Build history of the part. All positions in model axes, mm. A direction names the side the tool comes from. Coordinates: 2 decimals unless noted, no trailing zeros. Loops run counter-clockwise (first coordinate to the right, second up) from the corner with the lowest first, then second, coordinate; pieces in that order, holes last.
(1) Slice it at A-A (z = -1). Give the cut face in (x, y), and give its area (3 significant figures).
(2) Slice it at D-D (x = 10). Give the cut face in (y, z).
(3) Tool access for faces 1 (the face through (15, 2, -28)), 2 (the face through (20, 1, -11.25)), 3 (the face through (16.845, 4.522, -9.03)): list every direction of +Z, -Z, +X, -X, +Y, -Y with a clear straight run to the whole face (end or side of a thin tool).
(4) Two-plate mould, pull along X, no slides. Class faces 4 (the face through (-11.22, 2.74, -8.78)), 5 (the face through (22.25, 1, -9)), 6 (the face through (-16, 4, 11.25)): pulls with the +X half, pulls with the -X half, needs draft (parallel to the pull), parting line crosses it, or undercut.
(5) Wall check: L1, parallel to X at y = 3.55, z = -27.5; L2, parallel to X at y = 0.75, z = -18.5; L3, parallel to X at y = 4.25, z = -9. Give the ranges that are in metal, low to high.
(6) Slice it at B-B (y = 0.75). Give the cut face in (x, z), and give its area (4 significant figures).
(7) Flat gauge pins, fed straight in: P1, Ø1.5, axis at x = -13.5, y = 3.5, coming from the +Z side; P2, Ø2, axis at y = 2.5, z = -2, coming from the -X side; P3, Ø1.8, axis at x = 20, y = 1, coming from the -Z side; P4, Ø1.5, axis at x = 4, z = -8.5, coming from the +Y side. Where does each tip first touch, or does it go through?
(8) Slice it at C-C (x = -7.5). Give the cut face in (y, z).
from build123d import *

# Parameters (mm, degrees)
SKETCH_1_W          = 4
SKETCH_1_H          = 17.5
SKETCH_1_H_2        = 5
EXTRUDE_1_DEPTH     = 4
SKETCH_1_7_W        = 44.5
SKETCH_1_7_H        = 5
EXTRUDE_2_DEPTH     = 3.5
SKETCH_2_W          = 18.5
SKETCH_2_H          = 1.5
CUT_EXTRUDE_1_DEPTH = 32.89533665
SKETCH_2_3_W        = 2.5
SKETCH_2_3_H        = 1.5
EXTRUDE_4_DEPTH     = 22.5
FILLET_1_R          = 1
FILLET_2_R          = 1.5
FILLET_3_R          = 1
SKETCH_5_W          = 2.5
SKETCH_5_H          = 2
CUT_EXTRUDE_2_DEPTH = 43.315038698
SKETCH_10_R         = 0.4
CUT_EXTRUDE_3_DEPTH = 2


with BuildPart() as part:
    # 草图1 → 凸台-拉伸1 (new body)
    with BuildSketch(Plane(origin=(0, 0, 0), x_dir=(1, 0, 0), z_dir=(0, 1, 0))):
        with Locations((-15.75, -2.5)):
            Rectangle(SKETCH_1_W, SKETCH_1_H)
        with Locations((15.75, -2.5)):
            Rectangle(SKETCH_1_W, SKETCH_1_H)
        with Locations((15.75, 8.75)):
            Rectangle(SKETCH_1_W, SKETCH_1_H_2)
        with Locations((-15.75, 8.75)):
            Rectangle(SKETCH_1_W, SKETCH_1_H_2)
    extrude(amount=EXTRUDE_1_DEPTH)

    # 草图1<7> → 凸台-拉伸2 (add)
    with BuildSketch(Plane(origin=(0, 0, 0), x_dir=(1, 0, 0), z_dir=(0, 1, 0))):
        with Locations((0, 8.75)):
            Rectangle(SKETCH_1_7_W, SKETCH_1_7_H)
    extrude(amount=EXTRUDE_2_DEPTH)

    # 草图2 → 切除-拉伸1 (cut, through all)
    with BuildSketch(Plane(origin=(0, 0, -11.25), x_dir=(-1, 0, 0), z_dir=(0, 0, -1))):
        with Locations((0, 2.75)):
            Rectangle(SKETCH_2_W, SKETCH_2_H)
        Polygon((13.25, 3.5), (9.25, 3.5), (9.25, 2), align=None)
        Polygon((-9.25, 3.5), (-13.25, 3.5), (-9.25, 2), align=None)
        Polygon((-22.25, 3.5), (-22.25, 2), (-18.25, 3.5), align=None)
        Polygon((22.25, 3.5), (18.25, 3.5), (22.25, 2), align=None)
    extrude(amount=-CUT_EXTRUDE_1_DEPTH, mode=Mode.SUBTRACT)

    # 草图2<3> → 凸台-拉伸4 (add, through all)
    with BuildSketch(Plane(origin=(0, 0, -11.25), x_dir=(-1, 0, 0), z_dir=(0, 0, -1))):
        with Locations((-15.75, 7.25)):
            Rectangle(SKETCH_2_3_W, SKETCH_2_3_H)
        Polygon((-15, 6.5), (-16.5, 6.5), (-16.5, 4), (-15.75, 4), (-15, 4), align=None)
        with Locations((15.75, 7.25)):
            Rectangle(SKETCH_2_3_W, SKETCH_2_3_H)
        Polygon((16.5, 6.5), (15, 6.5), (15, 4), (15.75, 4), (16.5, 4), align=None)
    extrude(amount=-EXTRUDE_4_DEPTH)

    # 圆角1
    # the kernel refuses this fillet: 1 mm, written as the material it adds along each edge
    with BuildSketch(Plane(origin=(-16.5, 6.5, -11.25), x_dir=(0, -1, 0), z_dir=(0, 0, 1))) as fillet_1_piece_1:
        with BuildLine():
            CenterArc((0.866025404, -1), FILLET_1_R, 90, 60)
            Line((0, -0.5), (-0.017320508, -0.49))
            ThreePointArc((-0.017320508, -0.49), (-0.02, -0.25), (-0.02, 0))
            Line((-0.02, 0), (0, 0.02))
            Line((0, 0.02), (0.866025404, 0.02))
            Line((0.866025404, 0.02), (0.866025404, 0))
        make_face()
    extrude(amount=22.5)
    with BuildSketch(Plane(origin=(-15, 6.5, -11.25), x_dir=(0, -1, 0), z_dir=(0, 0, 1)), Plane(origin=(16.5, 6.5, -11.25), x_dir=(0, -1, 0), z_dir=(0, 0, 1))) as fillet_1_piece_2:
        with BuildLine():
            CenterArc((0.866025404, 1), FILLET_1_R, 210, 60)
            Line((0, 0.5), (-0.017320508, 0.49))
            ThreePointArc((-0.017320508, 0.49), (-0.02, 0.25), (-0.02, 0))
            Line((-0.02, 0), (0, -0.02))
            Line((0, -0.02), (0.866025404, -0.02))
            Line((0.866025404, -0.02), (0.866025404, 0))
        make_face()
    extrude(amount=22.5)
    with BuildSketch(Plane(origin=(15, 6.5, -11.25), x_dir=(-1, 0, 0), z_dir=(0, 0, 1))) as fillet_1_piece_3:
        with BuildLine():
            CenterArc((1, 0.866025404), FILLET_1_R, 180, 60)
            Line((0, 0.866025404), (-0.02, 0.866025404))
            Line((-0.02, 0.866025404), (-0.02, 0))
            Line((-0.02, 0), (0, -0.02))
            ThreePointArc((0, -0.02), (0.25, -0.02), (0.49, -0.017320508))
            Line((0.49, -0.017320508), (0.5, 0))
        make_face()
    extrude(amount=22.5)

    # 圆角2
    # the kernel refuses this fillet: 1.5 mm, written as the material it adds along each edge
    with BuildSketch(Plane(origin=(16.5, 4, -11.25), x_dir=(1, 0, 0), z_dir=(0, 0, 1)), Plane(origin=(-15, 4, -11.25), x_dir=(1, 0, 0), z_dir=(0, 0, 1))) as fillet_2_piece_1:
        with BuildLine():
            CenterArc((1.5, 1.479019946), FILLET_2_R, 180, 80.405931773)
            Line((0, 1.479019946), (-0.03, 1.479019946))
            Line((-0.03, 1.479019946), (-0.03, 0))
            Line((-0.03, 0), (0, -0.03))
            ThreePointArc((0, -0.03), (0.625, -0.03), (1.245, -0.029580399))
            Line((1.245, -0.029580399), (1.25, 0))
        make_face()
    extrude(amount=22.5)
    with BuildSketch(Plane(origin=(15, 4, -11.25), x_dir=(0, 1, 0), z_dir=(0, 0, 1)), Plane(origin=(-16.5, 4, -11.25), x_dir=(0, 1, 0), z_dir=(0, 0, 1))) as fillet_2_piece_2:
        with BuildLine():
            CenterArc((1.479019946, 1.5), FILLET_2_R, 189.594068227, 80.405931773)
            Line((0, 1.25), (-0.029580399, 1.245))
            ThreePointArc((-0.029580399, 1.245), (-0.03, 0.625), (-0.03, 0))
            Line((-0.03, 0), (0, -0.03))
            Line((0, -0.03), (1.479019946, -0.03))
            Line((1.479019946, -0.03), (1.479019946, 0))
        make_face()
    extrude(amount=22.5)

    # 圆角3
    fillet_3_edges = [part.edges().sort_by_distance(p)[0] for p in [
        (14.5, 8, 0),
        (17, 8, 0),
        (-17, 8, 0),
        (-14.5, 8, 0),
    ]]
    fillet(fillet_3_edges, radius=FILLET_3_R)

    # 草图5 → 切除-拉伸2 (cut, through all)
    with BuildSketch(Plane(origin=(17.75, 0, 0), x_dir=(0, 0, -1), z_dir=(1, 0, 0))):
        with Locations((-10, 1)):
            Rectangle(SKETCH_5_W, SKETCH_5_H)
    extrude(amount=-CUT_EXTRUDE_2_DEPTH, mode=Mode.SUBTRACT)

    # 草图10 → 切除-拉伸3 (cut)
    with BuildSketch(Plane.XZ.offset(-2)):
        with Locations(Location((15.75, 10, 0), (0, 0, 270))):
            Circle(SKETCH_10_R)
        with Locations(Location((-15.75, 10, 0), (0, 0, 270))):
            Circle(SKETCH_10_R)
    extrude(amount=-CUT_EXTRUDE_3_DEPTH, mode=Mode.SUBTRACT)

    # 镜向1: part across plane


with BuildPart() as part_1:
    add(part.part)
    add(part.part.mirror(Plane(origin=(0, 0, -8.75), x_dir=(1, 0, 0), z_dir=(0, 0, -1))))


solid = part_1.part
Response values:
1. outline: (-17.75, 0) - (-13.75, 0) - (-13.75, 4) arc R1.5 cw to (-15, 5.48) - (-15, 5.63) arc R1 cw to (-14.5, 6.5) - (-14.5, 7) arc R1 ccw to (-15.5, 8) - (-16, 8) arc R1 ccw to (-17, 7) - (-17, 6.5) arc R1 cw to (-16.5, 5.63) - (-16.5, 5.48) arc R1.5 cw to (-17.75, 4) - close; (13.75, 0) - (17.75, 0) - (17.75, 4) arc R1.5 cw to (16.5, 5.48) - (16.5, 5.63) arc R1 cw to (17, 6.5) - (17, 7) arc R1 ccw to (16, 8) - (15.5, 8) arc R1 ccw to (14.5, 7) - (14.5, 6.5) arc R1 cw to (15, 5.63) - (15, 5.48) arc R1.5 cw to (13.75, 4) - close
1. area: 48.5 mm2
2. outline: (0, -11.25) - (2.28, -11.25) - (2.28, -6.25) - (0, -6.25) - close
3. face 1: -Z, +X, -X, -Y
3. face 2: -Z, +X, +Y, -Y
3. face 3: +Z, -Z, +X
4. face 4: undercut
4. face 5: pulls with the +X half
4. face 6: needs draft
5. L1: x = -17.75 to -16.15, -15.35 to -13.75, 13.75 to 15.35, 16.15 to 17.75
5. L2: x = -17.75 to -13.75, 13.75 to 17.75
5. L3: x = -17.14 to -14.36, 14.36 to 17.14
6. outline: (-22.25, -11.25) - (-17.75, -11.25) - (-17.75, -26.25) - (-13.75, -26.25) - (-13.75, -11.25) - (13.75, -11.25) - (13.75, -26.25) - (17.75, -26.25) - (17.75, -11.25) - (22.25, -11.25) - (22.25, -6.25) - (17.75, -6.25) - (17.75, 8.75) - (13.75, 8.75) - (13.75, -6.25) - (-13.75, -6.25) - (-13.75, 8.75) - (-17.75, 8.75) - (-17.75, -6.25) - (-22.25, -6.25) - close
6. area: 462.5 mm2
7. P1: stops at z = 11.25
7. P2: stops at x = -17.75
7. P3: stops at z = -11.25
7. P4: stops at y = 2
8. outline: (0, -11.25) - (2, -11.25) - (2, -6.25) - (0, -6.25) - close
